from build123d import *

# Parameters (mm, degrees)
BOSS_EXTRUDE1_DEPTH = 79
SKETCH2_W           = 38
SKETCH2_H           = 58
CUT_EXTRUDE1_DEPTH  = 79
SKETCH2_4_W         = 44
SKETCH2_4_H         = 64
SKETCH2_4_W_2       = 38
SKETCH2_4_H_2       = 58
BOSS_EXTRUDE2_DEPTH = 11.2
SKETCH3_W           = 4
SKETCH3_H           = 27.5
CUT_EXTRUDE2_DEPTH  = 11.2
SKETCH4_R           = 3.719736595
CUT_EXTRUDE3_DEPTH  = 11.2


with BuildPart() as part:
    # Sketch1 → Boss-Extrude1 (new body)
    with BuildSketch(Plane.XY):
        with BuildLine():
            add(Edge.make_bspline(
                [(-25.17005526, -15), (-24.97113304, -15.005772519), (-24.766780605, -15.005846852), (-24.556789143, -15)],
                knots=[0.971548373, 0.971548373, 0.971548373, 0.971548373, 1, 1, 1, 1], degree=3))
            add(Edge.make_bspline(
                [(-37, -5.5), (-33.438353398, -6.048030585), (-32.154131783, -11.961146854), (-27.991532312, -14.91812363), (-25.17005526, -15)],
                knots=[0, 0, 0, 0, 0.5679956, 0.971548373, 0.971548373, 0.971548373, 0.971548373], degree=3))
            Line((-37, -5.5), (-44.050427966, -5.5))
            Line((-44.050427966, -5.5), (-44.050427966, -9))
            Line((-44.050427966, -9), (-38.622212975, -9))
            add(Edge.make_bspline(
                [(-38.622212975, -9), (-37.013577383, -8.940166603), (-35.066707272, -10.728314314), (-32.367433587, -16.596409153), (-30.698617033, -18.287184956), (-25.17005526, -18.5)],
                knots=[0, 0, 0, 0, 0.269469322, 0.622038388, 1, 1, 1, 1], degree=3))
            Line((-25.17005526, -18.5), (0, -18.5))
            Line((0, -18.5), (0, -15))
            Line((0, -15), (-24.556789143, -15))
        make_face()
        with BuildLine():
            Line((24.556789143, -15), (0, -15))
            Line((0, -15), (0, -18.5))
            Line((0, -18.5), (25.17005526, -18.5))
            add(Edge.make_bspline(
                [(38.622212975, -9), (37.013577383, -8.940166603), (35.066707272, -10.728314314), (32.367433587, -16.596409153), (30.698617033, -18.287184956), (25.17005526, -18.5)],
                knots=[0, 0, 0, 0, 0.269469322, 0.622038388, 1, 1, 1, 1], degree=3))
            Line((38.622212975, -9), (44.050427966, -9))
            Line((44.050427966, -9), (44.050427966, -5.5))
            Line((44.050427966, -5.5), (37, -5.5))
            add(Edge.make_bspline(
                [(37, -5.5), (33.438353398, -6.048030585), (32.154131783, -11.961146854), (27.991532312, -14.91812363), (25.17005526, -15)],
                knots=[0, 0, 0, 0, 0.5679956, 0.971548373, 0.971548373, 0.971548373, 0.971548373], degree=3))
            add(Edge.make_bspline(
                [(25.17005526, -15), (24.97113304, -15.005772519), (24.766780605, -15.005846852), (24.556789143, -15)],
                knots=[0.971548373, 0.971548373, 0.971548373, 0.971548373, 1, 1, 1, 1], degree=3))
        make_face()
    extrude(amount=BOSS_EXTRUDE1_DEPTH)

    # Sketch2 → Cut-Extrude1 (cut)
    with BuildSketch(Plane.XZ.offset(18.5)):
        with Locations((0, 39.360513879)):
            Rectangle(SKETCH2_W, SKETCH2_H)
    extrude(amount=-CUT_EXTRUDE1_DEPTH, mode=Mode.SUBTRACT)

    # Sketch2_4 → Boss-Extrude2 (add)
    with BuildSketch(Plane.XZ.offset(18.5)):
        with Locations((0, 39.360513879)):
            Rectangle(SKETCH2_4_W, SKETCH2_4_H)
        with Locations((0, 39.360513879)):
            Rectangle(SKETCH2_4_W_2, SKETCH2_4_H_2, mode=Mode.SUBTRACT)
    extrude(amount=BOSS_EXTRUDE2_DEPTH)

    # Sketch3 → Cut-Extrude2 (cut)
    with BuildSketch(Plane.XZ.offset(9)):
        with Locations((40.622212975, 59.446790211)):
            Rectangle(SKETCH3_W, SKETCH3_H)
        with Locations((40.622212975, 19.553209789)):
            Rectangle(SKETCH3_W, SKETCH3_H)
    cut_extrude2 = extrude(amount=-CUT_EXTRUDE2_DEPTH, mode=Mode.SUBTRACT)

    # Sketch4 → Cut-Extrude3 (cut)
    with BuildSketch(Plane.ZY.offset(22)):
        with Locations((21.211295074, -29.7)):
            Circle(SKETCH4_R)
    extrude(amount=-CUT_EXTRUDE3_DEPTH, mode=Mode.SUBTRACT)

    # Mirror1: Cut-Extrude2 across plane
    add(cut_extrude2.mirror(Plane(origin=(0, 0, 0), x_dir=(0, 0, 1), z_dir=(1, 0, 0))), mode=Mode.SUBTRACT)


solid = part.part
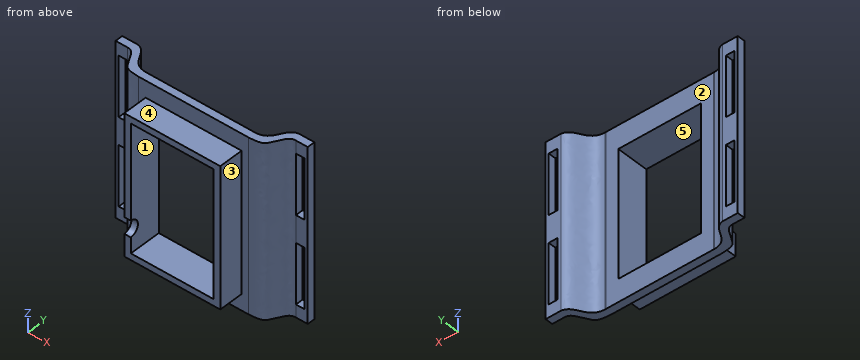
For this review, take the finished solid that the model builds, in its own axes (mm). Face numbers are marked on the shaded views. A direction names the side the tool comes from. Coordinates: 2 decimals unless noted, no trailing zeros. Loops run counter-clockwise (first coordinate to the right, second up) from the corner with the lowest first, then second, coordinate; pieces in that order, holes last. Notation, with made-up numbers: (-9.75, -34) - (45.25, -34) arc R27 cw to (45.25, 3) - close; hole circle Ø7 at (-13, 28.5). An arc over 180 degrees is marked (long way). Return JSON: item names as keys, results as strings.
Item 1: Take a section at B-B (y = -24). Give the boundary of the cut face in (x, z), then the cut area to 3 significant figures.
Determined:
{"outline": "(-22, 7.36) - (22, 7.36) - (22, 71.36) - (-22, 71.36) - close; hole (-19, 10.36) - (19, 10.36) - (19, 68.36) - (-19, 68.36) - close", "area": "612 mm2"}
Item 2: Take a section at C-C (x = 20.5). Give the boundary of the cut face in (y, z), then the cut area to 3 significant figures.
Determined:
{"outline": "(-29.7, 7.36) - (-18.5, 7.36) - (-18.5, 0) - (-15, 0) - (-15, 79) - (-18.5, 79) - (-18.5, 71.36) - (-29.7, 71.36) - close", "area": "993 mm2"}
Item 3: Mouldability with a two-part tool opening along X and no side actions: class the marked faces 3, 4 and 5 as pulls with the +X half, pulls with the -X half, needs draft (parallel to the pull), parting line crosses it, or undercut.
Determined:
{"face 3": "pulls with the +X half", "face 4": "needs draft", "face 5": "undercut"}
Item 4: For the marked faces 1 and 2, list the 3-axis set-ups (+Z, -Z, +X, -X, +Y, -Y) from which the entire face can be reached by the end or side of a thin tool; tool diameter is ignored.
Determined:
{"face 1": "+Y, -Y", "face 2": "+Z, -Z, +Y"}
Item 5: Insertion check: pin 1 (2.5 mm diameter, centred on x = -41.5, z = 39.5, fed in from -Y); pin 2 (1.5 mm diameter, centred on y = -24.5, z = 15.5, fed in from -X); pin 3 (9 mm diameter, centred on y = -21.5, z = 45.5, fed in from +X). Each pin has a flat end and moves straight along its axis. Give the tip position at first contact, or say it passes through.
Determined:
{"pin 1": "stops at y = -9", "pin 2": "stops at x = -22", "pin 3": "stops at x = 31.63"}
Item 6: Take a section at A-A (x = -17.5). Give the boundary of the cut face in (y, z), then the cut area to 3 significant figures.
Determined:
{"outline": "(-29.7, 7.36) - (-18.5, 7.36) - (-18.5, 0) - (-15, 0) - (-15, 10.36) - (-29.7, 10.36) - close; (-29.7, 68.36) - (-15, 68.36) - (-15, 79) - (-18.5, 79) - (-18.5, 71.36) - (-29.7, 71.36) - close", "area": "141 mm2"}
Item 7: For line 1 (Z direction, x = 12.5, y = -23.75); line 2 (X direction, y = -20.75, z = 11.5); line 3 (X direction, y = -7, z = 48.5), list the stretches that pass through material, from the lowest coordinate up.
Determined:
{"line 1": "z = 7.36 to 10.36, 68.36 to 71.36", "line 2": "x = -22 to -19, 19 to 22", "line 3": "x = -44.05 to -42.62, -38.62 to -34.11, 34.11 to 38.62, 42.62 to 44.05"}
Item 8: Take a section at D-D (z = 52.5). State how many separate pieces and enclosed holes the cut face has, then the cut area to 3 significant figures.
Determined:
{"separate pieces": "4", "enclosed holes": "0", "area": "246 mm2"}
